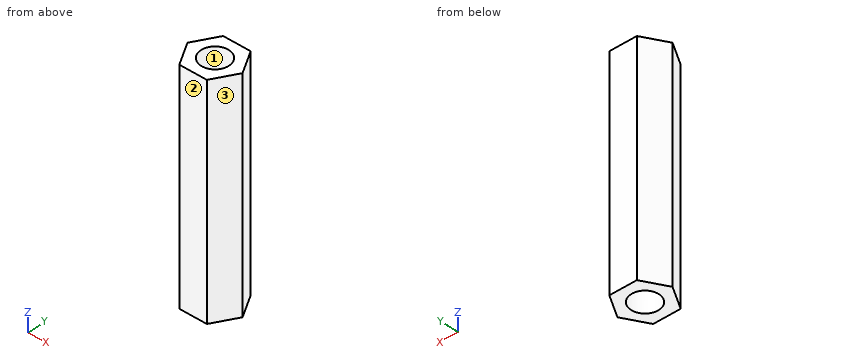
```python
from build123d import *

# Parameters (mm, degrees)
SKETCH1_R           = 1.397
BOSS_EXTRUDE1_DEPTH = 22.2758


with BuildPart() as part:
    # Sketch1 → Boss-Extrude1 (new body)
    with BuildSketch(Plane.XY):
        Polygon((2.62285315, 106.888971188), (1.259036344, 104.526771188), (2.62285315, 102.164571188), (5.350486762, 102.164571188), (6.714303568, 104.526771188), (5.350486762, 106.888971188), align=None)
        with Locations((3.986669956, 104.526771188)):
            Circle(SKETCH1_R, mode=Mode.SUBTRACT)
    extrude(amount=BOSS_EXTRUDE1_DEPTH)


solid = part.part
```
CAD build for the part. Positions are in the model's coordinates, mm. Face numbers are marked on the shaded views. Coordinates: 2 decimals unless noted, no trailing zeros. Order: outer loops, then holes, each group sorted by start corner. A loop starts at its lowest first (then second) coordinate and runs counter-clockwise, first axis right, second up. Notation, with made-up numbers: (0.25, 32) - (33.25, 32) arc R24 cw to (33.25, 52) - close; hole circle Ø10 at (-20, -17). An arc over 180 degrees is marked (long way). Use a Markdown table: item, result. Add a question column.
(1) Saw through at A-A (z = 20.5). Give the cut face in (x, y), then the cut area to 3 significant figures.
(2) Flat gauge pins, fed straight in: pin 1 (1.5 mm diameter, centred on y = 106.5, z = 13, fed in from -X); pin 2 (1.5 mm diameter, centred on y = 103, z = 6.5, fed in from +X). Where does each tip first touch, or does it go through?
(3) Saw through at D-D (y = 106.3). Give the cut face in (x, z).
(4) Saw through at C-C (y = 103.4). Give the cut face in (x, z).
(5) Drill centre lines: line 1 along Y through (x, z) = (4.65, 4.5); line 2 along Y through (x, z) = (2.8, 4); line 3 along X through (y, z) = (104.4, 21). Where is each one in solid material? Low to high. Write a range as [from, to].
(6) Saw through at B-B (x = 4.7). Give the cut face in (y, z).
(7) Pull direction X, two halves, no side cores. Call the marked faces 1, 2 and 3: +X half, -X half, draft (parallel to the pull), parting line (faces both ways), or undercut.
Solved:
| question | item | result |
|---|---|---|
| 1 | outline | (1.26, 104.53) - (2.62, 102.16) - (5.35, 102.16) - (6.71, 104.53) - (5.35, 106.89) - (2.62, 106.89) - close; hole circle Ø2.79 at (3.99, 104.53) |
| 1 | area | 13.2 mm² |
| 2 | pin 1 | stops at x = 1.97 |
| 2 | pin 2 | stops at x = 6.27 |
| 3 | outline | (2.28, 0) - (5.69, 0) - (5.69, 22.28) - (2.28, 22.28) - close |
| 4 | outline | (1.91, 0) - (3.16, 0) - (3.16, 22.28) - (1.91, 22.28) - close; (4.81, 0) - (6.06, 0) - (6.06, 22.28) - (4.81, 22.28) - close |
| 5 | line 1 | y = [102.16, 103.3], [105.76, 106.89] |
| 5 | line 2 | y = [102.16, 103.79], [105.26, 106.89] |
| 5 | line 3 | x = [1.33, 2.6], [5.38, 6.64] |
| 6 | outline | (102.16, 0) - (103.33, 0) - (103.33, 22.28) - (102.16, 22.28) - close; (105.73, 0) - (106.89, 0) - (106.89, 22.28) - (105.73, 22.28) - close |
| 7 | face 1 | undercut |
| 7 | face 2 | draft |
| 7 | face 3 | +X half |
